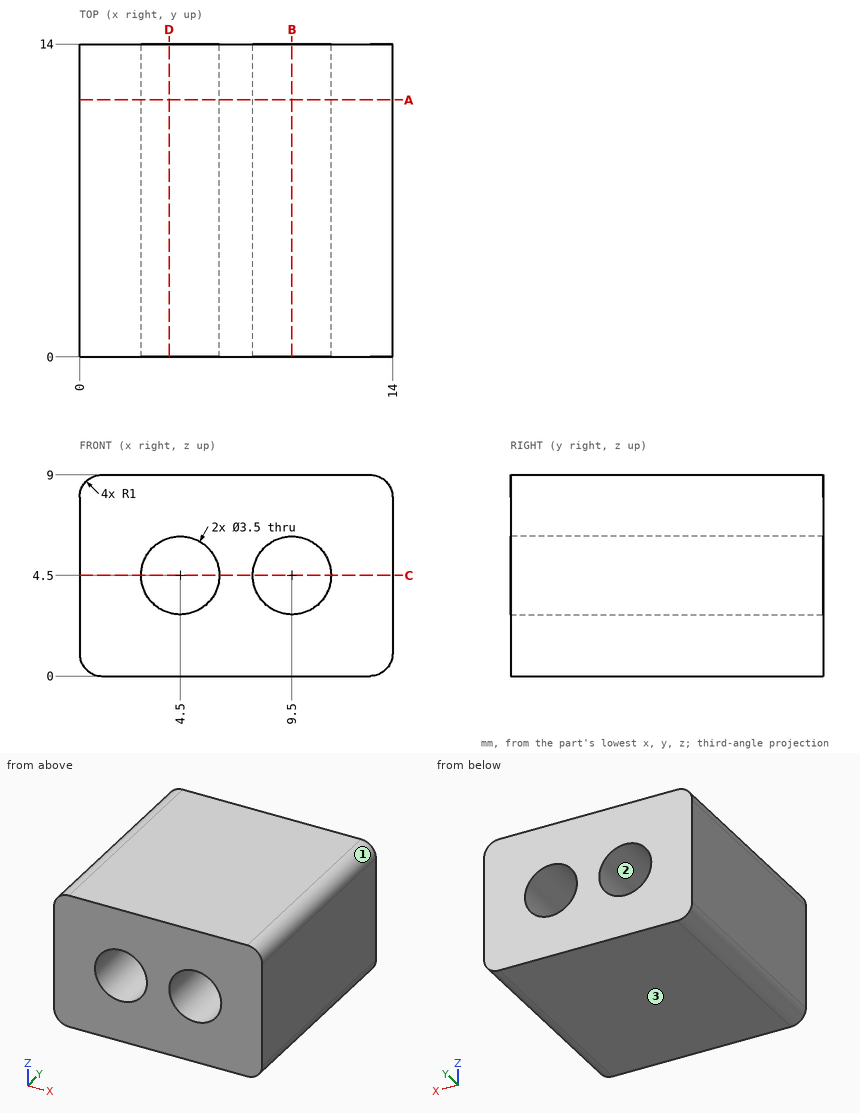
Job drawing, mm, ordinate dimensions from the low corner. One solid piece. Give positions to 0.01 mm unless a question says otherwise; leave off trailing zeros. Loops run counter-clockwise (first coordinate to the right, second up) from the corner with the lowest first, then second, coordinate; pieces in that order, holes last. Notation, with made-up numbers: M 60.5,2.5 L 100.5,2.5 A25 ccw 100.5,28.5 Z; hole C 41,9.5 d1. An arc over 180 degrees is marked long. Return JSON: item names as keys, results as strings.
1) Saw through at D-D, the plane x = 4. List the corners of the cut face in (y, z), then the cut area to 3 significant figures.
Calculated:
{"outline": "M 0,0 L 14,0 L 14,2.82 L 0,2.82 Z; M 0,6.18 L 14,6.18 L 14,9 L 0,9 Z", "area": "79.0 mm2"}
2) Pull direction Z, two halves, no side cores. Call the marked faces 1, 2 and 3: released by +Z, released by -Z, zero draft, split by the parting line, or undercut.
Calculated:
{"face 1": "released by +Z", "face 2": "undercut", "face 3": "released by -Z"}
3) Drill centre lines: line 1 (X direction, y = 3.5, z = 4.5); line 2 (Z direction, x = 4, y = 3.5); line 3 (Z direction, x = 3.75, y = 5.5). Where is each one in solid material? Low to high.
Calculated:
{"line 1": "x = 0 to 2.75, 6.25 to 7.75, 11.25 to 14", "line 2": "z = 0 to 2.82, 6.18 to 9", "line 3": "z = 0 to 2.92, 6.08 to 9"}
4) Saw through at C-C, the plane z = 4.5. List the corners of the cut face in (x, y).
Calculated:
{"outline": "M 0,0 L 2.75,0 L 2.75,14 L 0,14 Z; M 6.25,0 L 7.75,0 L 7.75,14 L 6.25,14 Z; M 11.25,0 L 14,0 L 14,14 L 11.25,14 Z"}
5) Saw through at A-A, the plane y = 11.5. List the corners of the cut face in (x, z), then the cut area to 3 significant figures.
Calculated:
{"outline": "M 0,1 A1 ccw 1,0 L 13,0 A1 ccw 14,1 L 14,8 A1 ccw 13,9 L 1,9 A1 ccw 0,8 Z; hole C 4.5,4.5 d3.5; hole C 9.5,4.5 d3.5", "area": "106 mm2"}
6) Saw through at B-B, the plane x = 9.5. List the corners of the cut face in (y, z).
Calculated:
{"outline": "M 0,0 L 14,0 L 14,2.75 L 0,2.75 Z; M 0,6.25 L 14,6.25 L 14,9 L 0,9 Z"}
